Input: part model. Units: mm. Frame: model coordinates. A direction names the side the tool comes from. Give positions to 0.01 mm unless a question says otherwise; leave off trailing zeros. Loops run counter-clockwise (first coordinate to the right, second up) from the corner with the lowest first, then second, coordinate; pieces in that order, holes last. Notation, with made-up numbers: M -13,2 L 16,2 A23 cw 16,17 Z; hole C 82.5,30.5 d8. An arc over 180 degrees is marked long. Use a Markdown table: item, result. Add a question column.
Autodesk Inventor part; units mm, degrees
ref_plane "YZ Plane" through (0, 0, 0) normal (1, 0, 0) x (0, 1, 0)
ref_plane "XZ Plane" through (0, 0, 0) normal (0, 1, 0) x (-1, 0, 0)
ref_plane "XY Plane" through (0, 0, 0) normal (0, 0, 1) x (1, 0, 0)
sketch "Sketch1" plane through (0, 0, 0) normal (0, 0, 1) x (1, 0, 0)
  circle A0 centre (0, 0) radius 63.5
  dimension "d0" = 127
extrude "Extrusion1" add sketch "Sketch1" against normal blind 101.6
sketch "Sketch2" plane through (0, 0, 0) normal (0, 0, 1) x (1, 0, 0)
  line L0 (-9.525, -31.75) -> (9.525, -31.75)
  line L1 (9.525, -31.75) -> (9.525, 31.75)
  line L2 (9.525, 31.75) -> (-9.525, 31.75)
  line L3 (-9.525, 31.75) -> (-9.525, -31.75)
  line L4 (-9.525, -31.75) -> (9.525, 31.75) construction
  line L5 (9.525, -31.75) -> (-9.525, 31.75) construction
  point P0 (0, 0)
  dimension "d3" = 63.5
  dimension "d4" = 19.05
extrude "Extrusion2" cut sketch "Sketch2" against normal blind 76.2
sketch "Sketch3" plane through (-9.525, -31.75, 0) normal (1, 0, 0) x (0, 0, -1)
  circle A0 centre (38.1, 31.75) radius 6.35
  line L0 (0, 0) -> (76.2, 0)
  line L1 (0, 0) -> (0, 63.5)
  point P0 (0, 31.75)
  dimension "d7" = 12.7
  dimension "d8" = 31.75
  dimension "d9" = 38.1
extrude "Extrusion3" cut sketch "Sketch3" along normal through all both and the other way through all
properties part number "CS-Slider"
1) Section query C-C, the plane x = 0. Return the cut outline in (y, z), and give its area (3 significant figures).
2) Contact query for flat-ended pins moving along their axis: P1, Ø1, axis at y = 26, z = -27, coming from the -X side; P2, Ø10, axis at y = 31.5, z = -44, coming from the +X side; P3, Ø10, axis at x = -9.5, z = -19, coming from the -Y side. Output: stop coordinate, or through.
3) Pull-direction query (Z, two-part tool) for faces 1 (the cylindrical face through (36.135, -0.279, -31.756)), 2 (the flat face through (-9.525, -7, -38)), 3 (the flat face through (13, 1, 0)); classes: pulls with the +Z half, pulls with the -Z half, needs draft (parallel to the pull), parting line crosses it, or undercut.
4) Ray query, line 1 (Z direction, x = 25, y = 0); line 2 (Y direction, x = 0, z = -57.5); line 3 (Y direction, x = 41, z = -38.1). Return the intervals inside material, ascending. Write a range as [from, to].
5) Section query D-D, the plane z = -60. Return the cut outline in (x, y) (3 decimals), and give its area (3 significant figures).
6) Reachability of faces 4 (the flat face through (0, -31.75, -38)), 5 (the flat face through (-1, 1, -101.6)) from +Z, -Z, +X, -X, +Y, -Y: full face, straight path, thin tool, end or side. Return the list, or none.
7) Section query B-B, the plane z = -38.1. Return the cut outline in (x, y) (3 decimals).
8) Section query A-A, the plane y = 0. Return the cut outline in (x, z) (3 decimals), and give its area (3 significant figures).
Entries:
| question | item | result |
|---|---|---|
| 1 | outline | M -63.5,-101.6 L 63.5,-101.6 L 63.5,0 L 31.75,0 L 31.75,-76.2 L -31.75,-76.2 L -31.75,0 L -63.5,0 Z |
| 1 | area | 8,060 mm² |
| 2 | P1 | stops at x = -58.15 |
| 2 | P2 | stops at x = 57.71 |
| 2 | P3 | stops at y = -63.34 |
| 3 | face 1 | undercut |
| 3 | face 2 | needs draft |
| 3 | face 3 | pulls with the +Z half |
| 4 | line 1 | z = [-101.6, -44.45], [-31.75, 0] |
| 4 | line 2 | y = [-63.5, -31.75], [31.75, 63.5] |
| 4 | line 3 | y = [-48.49, -6.35], [6.35, 48.49] |
| 5 | outline | C 0,0 d127; hole M -9.525,-31.75 L 9.525,-31.75 L 9.525,31.75 L -9.525,31.75 Z |
| 5 | area | 11,500 mm² |
| 6 | face 4 | +Z |
| 6 | face 5 | -Z, +X, -X, +Y, -Y |
| 7 | outline | M -63.182,-6.35 A63.5 ccw 63.182,-6.35 L 9.525,-6.35 L 9.525,-31.75 L -9.525,-31.75 L -9.525,-6.35 Z; M -63.182,6.35 L -9.525,6.35 L -9.525,31.75 L 9.525,31.75 L 9.525,6.35 L 63.182,6.35 A63.5 ccw Z |
| 8 | outline | M -63.5,-101.6 L 63.5,-101.6 L 63.5,-44.45 L 9.525,-44.45 L 9.525,-76.2 L -9.525,-76.2 L -9.525,-44.45 L -63.5,-44.45 Z; M -63.5,-31.75 L -9.525,-31.75 L -9.525,0 L -63.5,0 Z; M 9.525,-31.75 L 63.5,-31.75 L 63.5,0 L 9.525,0 Z |
| 8 | area | 10,100 mm² |
